```python
from build123d import *

# Parameters (mm, degrees)
F2_SIZE = 0.5
F3_R    = 0.15


with BuildPart() as f1:
    # F0 (on Right) → F1 (revolve)
    with BuildSketch(Plane.YZ):
        Polygon((3, 1), (3, 0), (4, 0), (4, 2), (2.5, 2), (2.5, 7.394109), (1.5, 7.662058), (2.5, 8.239408), (2.5, 8.627035), (0, 8.627035), (0, 1), align=None)
    revolve(axis=Axis((0, 0, 18.218487), (0, 0, 1)))

    # F2
    f2_edges = [f1.edges().sort_by_distance(p)[0] for p in [
        (0, -2.5, 2),
        (0, -3, 1),
    ]]
    chamfer(f2_edges, length=F2_SIZE)

    # F3
    f3_edges = [f1.edges().sort_by_distance(p)[0] for p in [
        (0, -1.5, 7.662058),
    ]]
    fillet(f3_edges, radius=F3_R)


solid = f1.part
```
The listing builds one solid part. Answer for the finished solid, in the listing's coordinates (mm). A direction names the side the tool comes from. Round coordinates to 2 decimals unless told otherwise and drop trailing zeros. Loops run counter-clockwise (first coordinate to the right, second up) from the corner with the lowest first, then second, coordinate; pieces in that order, holes last. Notation, with made-up numbers: (2.5, 53.25) -> (57.5, 53.25) arc R13 ccw to (57.5, 67.25) -> close; hole circle Ø6 at (41.5, -17.75). An arc over 180 degrees is marked (long way). Use one line per item in the form item = value.
1. The part is cut by section B-B on x = -3.5. Determine the outline of the cut face in (y, z), and give its area (3 significant figures).
Answer key:
outline = (-1.94, 0) -> (1.94, 0) -> (1.94, 2) -> (-1.94, 2) -> close
area = 7.75 mm²
2. The part is cut by section A-A on z = 5.5. Determine the outline of the cut face in (x, y), and give its area (3 significant figures).
Answer key:
outline = circle Ø5 at (0, 0)
area = 19.6 mm²
3. For a pull along X with two mould halves and no side action, classify faces 1 (the flat face through (-3, -1, 0)), 2 (the cylindrical face through (2.44, -0.54, 4.98)), 3 (the cylindrical face through (-0.1, -3, 0.2)) as released by +X, released by -X, zero draft, split by the parting line, or undercut.
Answer key:
face_1 = zero draft
face_2 = split by the parting line
face_3 = undercut
4. Flat-ended cylindrical pins translate along their axes: pin 1 Ø1 at (x, y) = (0.5, 3) entering from +Z; pin 2 Ø2 at (x, z) = (-1, 1.5) entering from +Y; pin 3 Ø4 at (x, y) = (0, 0) entering from -Z. Find the tip coordinate at first contact, or state that the pin passes through.
Answer key:
pin_1 = 2.46
pin_2 = 4
pin_3 = 1
5. A tool of negligible diameter and unlimited length cuts with its end or side. For faces 4 (the flat face through (0, 0, 1)), 5 (the flat face through (0, 0, 8.627)), 6 (the cylindrical face through (2.44, -0.54, 8.44)), from which of +Z, -Z, +X, -X, +Y, -Y can it reach the whole face along a straight path? Write none if from no direction.
Answer key:
face_4 = -Z
face_5 = +Z, +X, -X, +Y, -Y
face_6 = +Z
6. Find the intervals of material crossed by probe 1 along X at (y, z) = (0, 0.45); probe 2 along Z at (x, y) = (0.5, 3), in increasing order. Write a range as [from, to].
Answer key:
probe_1 = [-4, -3], [3, 4]
probe_2 = [0, 2]
7. The part is cut by section C-C on x = 3.25. Determine the outline of the cut face in (y, z).
Answer key:
outline = (-2.33, 0) -> (2.33, 0) -> (2.33, 2) -> (-2.33, 2) -> close
